from build123d import *

# Parameters (mm, degrees)
SKETCH1_W           = 27.31
SKETCH1_H           = 7.62
SKETCH1_R           = 1.22
BOSS_EXTRUDE1_DEPTH = 4.24
BOSS_EXTRUDE2_DEPTH = 8.89


with BuildPart() as part:
    # Sketch1 → Boss-Extrude1 (new body)
    # profile 1 of 9: a face of its own
    with BuildSketch(Plane(origin=(0, 0, 0), x_dir=(1, 0, 0), z_dir=(0, 1, 0))):
        with Locations((13.655, -3.81)):
            Rectangle(SKETCH1_W, SKETCH1_H)
        with Locations(Location((2.67, -3.81, 0), (0, 0, 270))):
            Circle(SKETCH1_R, mode=Mode.SUBTRACT)
        with BuildLine():
            ThreePointArc((20.540684506, -5.56), (19.966861952, -5.9629153), (19.28025799, -6.105))
            Line((19.28025799, -6.105), (8.04147976, -6.105))
            ThreePointArc((8.04147976, -6.105), (7.354875799, -5.9629153), (6.781053245, -5.56))
            Line((6.781053245, -5.56), (5.605, -5.56))
            Line((5.605, -5.56), (5.605, -3.575873574))
            ThreePointArc((5.605, -3.575873574), (5.51591253, -3.266011562), (5.485868875, -2.945))
            ThreePointArc((5.485868875, -2.945), (5.51591253, -2.623988438), (5.605, -2.314126426))
            Line((5.605, -2.314126426), (5.605, -2.06))
            Line((5.605, -2.06), (5.729371314, -2.06))
            ThreePointArc((5.729371314, -2.06), (6.360927357, -1.44101363), (7.215868875, -1.215))
            Line((7.215868875, -1.215), (20.105868875, -1.215))
            ThreePointArc((20.105868875, -1.215), (20.960810394, -1.44101363), (21.592366437, -2.06))
            Line((21.592366437, -2.06), (21.705, -2.06))
            Line((21.705, -2.06), (21.705, -2.284939665))
            ThreePointArc((21.705, -2.284939665), (21.835868875, -2.945), (21.705, -3.605060335))
            Line((21.705, -3.605060335), (21.705, -5.56))
            Line((21.705, -5.56), (20.540684506, -5.56))
        make_face(mode=Mode.SUBTRACT)
        with Locations(Location((24.64, -3.81, 0), (0, 0, 270))):
            Circle(SKETCH1_R, mode=Mode.SUBTRACT)
    # profile 2 of 9: a face of its own
    with BuildSketch(Plane(origin=(0, 0, 0), x_dir=(1, 0, 0), z_dir=(0, 1, 0))):
        with BuildLine():
            Line((5.605, -5.56), (6.781053245, -5.56))
            ThreePointArc((6.781053245, -5.56), (6.652905637, -5.406873008), (6.543255812, -5.24))
            Line((6.543255812, -5.24), (5.717644927, -3.81))
            ThreePointArc((5.717644927, -3.81), (5.656921043, -3.695054436), (5.605, -3.575873574))
            Line((5.605, -3.575873574), (5.605, -5.56))
        make_face()
    # profile 3 of 9: a face of its own
    with BuildSketch(Plane(origin=(0, 0, 0), x_dir=(1, 0, 0), z_dir=(0, 1, 0))):
        with BuildLine():
            Line((8.04147976, -6.105), (19.28025799, -6.105))
            ThreePointArc((19.28025799, -6.105), (19.966861952, -5.9629153), (20.540684506, -5.56))
            Line((20.540684506, -5.56), (6.781053245, -5.56))
            ThreePointArc((6.781053245, -5.56), (7.354875799, -5.9629153), (8.04147976, -6.105))
        make_face()
    # profile 4 of 9: a face of its own
    with BuildSketch(Plane(origin=(0, 0, 0), x_dir=(1, 0, 0), z_dir=(0, 1, 0))):
        with BuildLine():
            Line((5.729371314, -2.06), (21.592366437, -2.06))
            ThreePointArc((21.592366437, -2.06), (20.960810394, -1.44101363), (20.105868875, -1.215))
            Line((20.105868875, -1.215), (7.215868875, -1.215))
            ThreePointArc((7.215868875, -1.215), (6.360927357, -1.44101363), (5.729371314, -2.06))
        make_face()
    # profile 5 of 9: a face of its own
    with BuildSketch(Plane(origin=(0, 0, 0), x_dir=(1, 0, 0), z_dir=(0, 1, 0))):
        with BuildLine():
            ThreePointArc((20.778481939, -5.24), (20.668832114, -5.406873008), (20.540684506, -5.56))
            Line((20.540684506, -5.56), (21.705, -5.56))
            Line((21.705, -5.56), (21.705, -3.605060335))
            ThreePointArc((21.705, -3.605060335), (21.65793272, -3.709197501), (21.604092824, -3.81))
            Line((21.604092824, -3.81), (20.778481939, -5.24))
        make_face()
    # profile 6 of 9: a face of its own
    with BuildSketch(Plane(origin=(0, 0, 0), x_dir=(1, 0, 0), z_dir=(0, 1, 0))):
        with BuildLine():
            Line((21.705, -2.284939665), (21.705, -3.605060335))
            ThreePointArc((21.705, -3.605060335), (21.835868875, -2.945), (21.705, -2.284939665))
        make_face()
    # profile 7 of 9: a face of its own
    with BuildSketch(Plane(origin=(0, 0, 0), x_dir=(1, 0, 0), z_dir=(0, 1, 0))):
        with BuildLine():
            ThreePointArc((5.485868875, -2.945), (5.51591253, -3.266011562), (5.605, -3.575873574))
            Line((5.605, -3.575873574), (5.605, -2.314126426))
            ThreePointArc((5.605, -2.314126426), (5.51591253, -2.623988438), (5.485868875, -2.945))
        make_face()
    # profile 8 of 9: a face of its own
    with BuildSketch(Plane(origin=(0, 0, 0), x_dir=(1, 0, 0), z_dir=(0, 1, 0))):
        with BuildLine():
            Line((5.605, -2.06), (5.605, -2.314126426))
            ThreePointArc((5.605, -2.314126426), (5.661981888, -2.184516451), (5.729371314, -2.06))
            Line((5.729371314, -2.06), (5.605, -2.06))
        make_face()
    # profile 9 of 9: a face of its own
    with BuildSketch(Plane(origin=(0, 0, 0), x_dir=(1, 0, 0), z_dir=(0, 1, 0))):
        with BuildLine():
            ThreePointArc((21.592366437, -2.06), (21.652777263, -2.17041983), (21.705, -2.284939665))
            Line((21.705, -2.284939665), (21.705, -2.06))
            Line((21.705, -2.06), (21.592366437, -2.06))
        make_face()
    extrude(amount=BOSS_EXTRUDE1_DEPTH)

    # Sketch1_2 → Boss-Extrude2 (add)
    with BuildSketch(Plane(origin=(0, 0, 0), x_dir=(1, 0, 0), z_dir=(0, 1, 0))):
        with BuildLine():
            Line((5.729371314, -2.06), (21.592366437, -2.06))
            ThreePointArc((21.592366437, -2.06), (20.960810394, -1.44101363), (20.105868875, -1.215))
            Line((20.105868875, -1.215), (7.215868875, -1.215))
            ThreePointArc((7.215868875, -1.215), (6.360927357, -1.44101363), (5.729371314, -2.06))
        make_face()
        with BuildLine():
            Line((8.04147976, -6.105), (19.28025799, -6.105))
            ThreePointArc((19.28025799, -6.105), (19.966861952, -5.9629153), (20.540684506, -5.56))
            Line((20.540684506, -5.56), (6.781053245, -5.56))
            ThreePointArc((6.781053245, -5.56), (7.354875799, -5.9629153), (8.04147976, -6.105))
        make_face()
        with BuildLine():
            Line((6.781053245, -5.56), (20.540684506, -5.56))
            ThreePointArc((20.540684506, -5.56), (20.668832114, -5.406873008), (20.778481939, -5.24))
            Line((20.778481939, -5.24), (21.604092824, -3.81))
            ThreePointArc((21.604092824, -3.81), (21.65793272, -3.709197501), (21.705, -3.605060335))
            Line((21.705, -3.605060335), (21.705, -2.284939665))
            ThreePointArc((21.705, -2.284939665), (21.652777263, -2.17041983), (21.592366437, -2.06))
            Line((21.592366437, -2.06), (5.729371314, -2.06))
            ThreePointArc((5.729371314, -2.06), (5.661981888, -2.184516451), (5.605, -2.314126426))
            Line((5.605, -2.314126426), (5.605, -3.575873574))
            ThreePointArc((5.605, -3.575873574), (5.656921043, -3.695054436), (5.717644927, -3.81))
            Line((5.717644927, -3.81), (6.543255812, -5.24))
            ThreePointArc((6.543255812, -5.24), (6.652905637, -5.406873008), (6.781053245, -5.56))
        make_face()
        with BuildLine():
            ThreePointArc((5.485868875, -2.945), (5.51591253, -3.266011562), (5.605, -3.575873574))
            Line((5.605, -3.575873574), (5.605, -2.314126426))
            ThreePointArc((5.605, -2.314126426), (5.51591253, -2.623988438), (5.485868875, -2.945))
        make_face()
        with BuildLine():
            Line((21.705, -2.284939665), (21.705, -3.605060335))
            ThreePointArc((21.705, -3.605060335), (21.835868875, -2.945), (21.705, -2.284939665))
        make_face()
    extrude(amount=BOSS_EXTRUDE2_DEPTH)


solid = part.part
The model under review builds one solid part; all positions refer to its coordinate system, in mm. A direction names the side the tool comes from. Give positions to 0.01 mm unless a question says otherwise; leave off trailing zeros. Loops run counter-clockwise (first coordinate to the right, second up) from the corner with the lowest first, then second, coordinate; pieces in that order, holes last. Notation, with made-up numbers: (13, -12.75) -> (65, -12.75) arc R25 cw to (65, 16.25) -> close; hole circle Ø7 at (25, 7). An arc over 180 degrees is marked (long way). Write each question's results on one line, items separated by ' | '.
1) Take a section at D-D, the plane x = 8.5. Give the boundary of the cut face in (y, z) (3 decimals), plus the area to 3 significant figures.
Conclusion:
outline: (0, 0) -> (4.24, 0) -> (4.24, 1.215) -> (8.89, 1.215) -> (8.89, 6.105) -> (4.24, 6.105) -> (4.24, 7.62) -> (0, 7.62) -> close | area: 55.0 mm^2
2) Take a section at C-C, the plane y = 7. Give the boundary of the cut face in (x, z) (3 decimals), plus the area to 3 significant figures.
Conclusion:
outline: (5.718, 3.81) arc R1.73 ccw to (7.216, 1.215) -> (20.106, 1.215) arc R1.73 ccw to (21.604, 3.81) -> (20.778, 5.24) arc R1.73 ccw to (19.28, 6.105) -> (8.041, 6.105) arc R1.73 ccw to (6.543, 5.24) -> close | area: 74.1 mm^2
3) Take a section at B-B, the plane z = 3.25. Give the boundary of the cut face in (x, y), plus the area to 3 significant figures.
Conclusion:
outline: (0, 0) -> (1.59, 0) -> (1.59, 4.24) -> (0, 4.24) -> close; (3.75, 0) -> (23.56, 0) -> (23.56, 4.24) -> (21.81, 4.24) -> (21.81, 8.89) -> (5.51, 8.89) -> (5.51, 4.24) -> (3.75, 4.24) -> close; (25.72, 0) -> (27.31, 0) -> (27.31, 4.24) -> (25.72, 4.24) -> close | area: 173 mm^2
4) Insertion check: pin 1 Ø1.4 at (x, y) = (14, 5.5) entering from +Z (3 decimals); pin 2 Ø3 at (x, z) = (2.67, 3.81) entering from +Y; pin 3 Ø1 at (x, y) = (11, 6.5) entering from -Z (3 decimals). Each pin has a flat end and moves straight along its axis. Give the tip position at first contact, or say it passes through.
Conclusion:
pin 1: stops at z = 6.105 | pin 2: stops at y = 4.24 | pin 3: stops at z = 1.215
5) Take a section at A-A, the plane x = 2.67. Give the boundary of the cut face in (y, z), plus the area to 3 significant figures.
Conclusion:
outline: (0, 0) -> (4.24, 0) -> (4.24, 2.59) -> (0, 2.59) -> close; (0, 5.03) -> (4.24, 5.03) -> (4.24, 7.62) -> (0, 7.62) -> close | area: 22.0 mm^2
6) For line 1 along X through (y, z) = (1.2, 3.81); line 2 along Z through (x, y) = (2.75, 3.5); line 3 along X through (y, z) = (3.5, 3), list the stretches that pass through material, from the lowest coordinate up. Write a range as from..to.
Conclusion:
line 1: x = 0..1.45, 3.89..23.42, 25.86..27.31 | line 2: z = 0..2.59, 5.03..7.62 | line 3: x = 0..1.76, 3.58..23.73, 25.55..27.31
7) Tool access review of faces 4 (the face through (14, 7, 6.105)), 5 (the face through (24.69, 2.09, 2.59)), 6 (the face through (21.186, 6.532, 4.535)), 7 (the face through (6.12, 6.53, 4.51)), 8 (the face through (14, 7, 1.215)): name each direction out of +Z, -Z, +X, -X, +Y, -Y from which nothing blocks a thin tool from reaching the whole face with its end or side.
Conclusion:
face 4: +Z, +X, -X, +Y | face 5: +Y, -Y | face 6: +Z, +X, +Y | face 7: +Z, -X, +Y | face 8: -Z, +X, -X, +Y
8) Draft analysis for pull direction X (two halves, no side actions). For faces 1 (the face through (13, 0, 4)), 2 (the face through (0, 2, 4)), 3 (the face through (3.495, 2.09, 2.911)), state which applies: pulls with the +X half, pulls with the -X half, needs draft (parallel to the pull), parting line crosses it, or undercut.
Conclusion:
face 1: needs draft | face 2: pulls with the -X half | face 3: undercut
